from build123d import *

# Parameters (mm, degrees)
ESTRUSIONE_ESTRUSIONE1_DEPTH = 37
SCHIZZO4_R                   = 8
TAGLIO_ESTRUSIONE1_DEPTH     = 44.794976881
RACCORDO1_R                  = 0.2


with BuildPart() as part:
    # Schizzo1 → Estrusione-Estrusione1 (new body)
    with BuildSketch(Plane(origin=(0, 0, 0), x_dir=(1, 0, 0), z_dir=(0, 1, 0))):
        Polygon((-15, 0), (15, 0), (15, -3), (12, -3), (12, -18), (-12, -18), (-12, -3), (-15, -3), align=None)
    extrude(amount=ESTRUSIONE_ESTRUSIONE1_DEPTH)

    # Schizzo4 → Taglio-Estrusione1 (cut, through all)
    with BuildSketch(Plane.XY.offset(18)):
        with Locations((0, 11)):
            Circle(SCHIZZO4_R)
    extrude(amount=-TAGLIO_ESTRUSIONE1_DEPTH, mode=Mode.SUBTRACT)

    # Raccordo1
    raccordo1_edges = [part.edges().sort_by_distance(p)[0] for p in [
        (12, 18.5, 3),
        (-12, 18.5, 3),
    ]]
    fillet(raccordo1_edges, radius=RACCORDO1_R)


solid = part.part
Can you work these out from the model? Positions are in its coordinate system, mm. A direction names the side the tool comes from. Coordinates: 2 decimals unless noted, no trailing zeros. Order: outer loops, then holes, each group sorted by start corner. A loop starts at its lowest first (then second) coordinate and runs counter-clockwise, first axis right, second up. Notation, with made-up numbers: (-9.5, 41.5) - (32.5, 41.5) arc R23 ccw to (32.5, 56.5) - close; hole circle Ø2 at (-16.75, 22). An arc over 180 degrees is marked (long way). Answer as a JSON object with one key per item and string values. Group by question number.
Q1. Imagine slicing it at C-C (z = 7.5). Please give me the cut outline in (x, y), and give its area (3 significant figures).
Q2. We'd pull the mould along X, two halves only. Please class faces 1 (the face through (-1.73, 3.19, 9.13)), 2 (the face through (0, 0, 9)), 3 (the face through (12, 18, 10)): +X half, -X half, draft (parallel to the pull), parting line (faces both ways), or undercut.
Q3. I need wall thicknesses on line 1 (Y direction, x = 0.25, z = 10); line 2 (Z direction, x = 13.75, y = 12.5); line 3 (X direction, y = 29.5, z = 8.75). Which ranges of each line are inside material? Lowest first, please. Write a range as from..to.
Q4. Imagine slicing it at D-D (y = 30). Please give me the cut outline in (x, z).
Q5. Imagine slicing it at A-A (x = 0). Please give me the cut outline in (y, z).
Q6. Will these pins go through, and if not, where does the flat tip stop? P1, Ø4.5, axis at y = 22.5, z = 13, coming from the -X side; P2, Ø0.8, axis at x = -13.5, y = 24.5, coming from the +Z side; P3, Ø13, axis at x = 0, y = 11, coming from the +Z side; P4, Ø4.5, axis at y = 22, z = 9.5, coming from the +X side.
Q7. Imagine slicing it at B-B (y = 11). Please give me the cut outline in (x, z).
Q8. On a 3-axis mill with a long thin cutter (end or side, diameter ignored), from which of +Z, -Z, +X, -X, +Y, -Y can I reach the whole of each face in a straight line? I mean faces 4 (the face through (0, 22, 0)), 5 (the face through (14, 18, 3)), 6 (the face through (-14, 18, 3)). Say none if no direction works.
Determined:
{
 "1": {"outline": "(-12, 0) - (12, 0) - (12, 37) - (-12, 37) - close; hole circle Ø16 at (0, 11)", "area": "687 mm2"},
 "2": {"face 1": "undercut", "face 2": "draft", "face 3": "+X half"},
 "3": {"line 1": "y = 0..3, 19..37", "line 2": "z = 0..3", "line 3": "x = -12..12"},
 "4": {"outline": "(-15, 0) - (15, 0) - (15, 3) - (12.2, 3) arc R0.2 cw to (12, 3.2) - (12, 18) - (-12, 18) - (-12, 3.2) arc R0.2 cw to (-12.2, 3) - (-15, 3) - close"},
 "5": {"outline": "(0, 0) - (3, 0) - (3, 18) - (0, 18) - close; (19, 0) - (37, 0) - (37, 18) - (19, 18) - close"},
 "6": {"P1": "stops at x = -12", "P2": "stops at z = 3", "P3": "passes through", "P4": "stops at x = 12"},
 "7": {"outline": "(-15, 0) - (-8, 0) - (-8, 18) - (-12, 18) - (-12, 3.2) arc R0.2 cw to (-12.2, 3) - (-15, 3) - close; (8, 0) - (15, 0) - (15, 3) - (12.2, 3) arc R0.2 cw to (12, 3.2) - (12, 18) - (8, 18) - close"},
 "8": {"face 4": "-Z, +X, -X, +Y, -Y", "face 5": "+Z, +X, +Y, -Y", "face 6": "+Z, -X, +Y, -Y"}
}
